```python
from build123d import *

# Parameters (mm, degrees)
F0_R     = 5
F0_R_2   = 4
F0_R_3   = 2.1
F1_DEPTH = 8
F2_DEPTH = 25
F3_R     = 4
F3_R_2   = 2.1
F4_DEPTH = 4
F5_DEPTH = 6
F6_DEPTH = 1
F7_R     = 0.5


with BuildPart() as f1:
    # F0 (on Top) → F1 (new body)
    with BuildSketch(Plane.XY):
        with BuildLine():
            ThreePointArc((-96.161356, -13.406398), (-102.161356, -19.406398), (-96.161356, -25.406398))
            Line((-96.161356, -25.406398), (-46.161356, -25.406398))
            ThreePointArc((-46.161356, -25.406398), (-40.161356, -19.406398), (-46.161356, -13.406398))
            Line((-46.161356, -13.406398), (-96.161356, -13.406398))
        make_face()
        with BuildLine():
            Line((-96.161356, -13.906398), (-46.161356, -13.906398))
            ThreePointArc((-46.161356, -13.906398), (-40.661356, -19.406398), (-46.161356, -24.906398))
            Line((-46.161356, -24.906398), (-96.161356, -24.906398))
            ThreePointArc((-96.161356, -24.906398), (-101.661356, -19.406398), (-96.161356, -13.906398))
        make_face(mode=Mode.SUBTRACT)
        with BuildLine():
            ThreePointArc((-46.161356, -24.906398), (-40.661356, -19.406398), (-46.161356, -13.906398))
            Line((-46.161356, -13.906398), (-96.161356, -13.906398))
            ThreePointArc((-96.161356, -13.906398), (-101.661356, -19.406398), (-96.161356, -24.906398))
            Line((-96.161356, -24.906398), (-46.161356, -24.906398))
        make_face()
        with Locations((-96.161356, -19.406398)):
            Circle(F0_R, mode=Mode.SUBTRACT)
        with BuildLine():
            ThreePointArc((-85.161356, -22.406398), (-88.161356, -19.406398), (-85.161356, -16.406398))
            Line((-85.161356, -16.406398), (-57.161356, -16.406398))
            ThreePointArc((-57.161356, -16.406398), (-54.161356, -19.406398), (-57.161356, -22.406398))
            Line((-57.161356, -22.406398), (-85.161356, -22.406398))
        make_face(mode=Mode.SUBTRACT)
        with Locations((-46.161356, -19.406398)):
            Circle(F0_R, mode=Mode.SUBTRACT)
        with Locations((-96.161356, -19.406398)):
            Circle(F0_R)
        with Locations((-96.161356, -19.406398)):
            Circle(F0_R_2, mode=Mode.SUBTRACT)
        with Locations((-96.161356, -19.406398)):
            Circle(F0_R_2)
        with Locations((-96.161356, -19.406398)):
            Circle(F0_R_3, mode=Mode.SUBTRACT)
        with Locations((-96.161356, -19.406398)):
            Circle(F0_R_3)
        with BuildLine():
            Line((-57.161356, -16.406398), (-85.161356, -16.406398))
            ThreePointArc((-85.161356, -16.406398), (-88.161356, -19.406398), (-85.161356, -22.406398))
            Line((-85.161356, -22.406398), (-57.161356, -22.406398))
            ThreePointArc((-57.161356, -22.406398), (-54.161356, -19.406398), (-57.161356, -16.406398))
        make_face()
        with Locations((-46.161356, -19.406398)):
            Circle(F0_R)
        with Locations((-46.161356, -19.406398)):
            Circle(F0_R_2, mode=Mode.SUBTRACT)
        with Locations((-46.161356, -19.406398)):
            Circle(F0_R_2)
        with Locations((-46.161356, -19.406398)):
            Circle(F0_R_3, mode=Mode.SUBTRACT)
        with Locations((-46.161356, -19.406398)):
            Circle(F0_R_3)
    extrude(amount=F1_DEPTH)

    # F0 (on Top) → F2 (cut)
    with BuildSketch(Plane.XY):
        with Locations((-96.161356, -19.406398)):
            Circle(F0_R_3)
        with Locations((-46.161356, -19.406398)):
            Circle(F0_R_3)
    extrude(amount=F2_DEPTH, mode=Mode.SUBTRACT)

    # F3 (on face) → F4 (cut)
    with BuildSketch(Plane.XY.offset(8)):
        with Locations((-96.161356, -19.406398)):
            Circle(F3_R)
        with Locations((-96.161356, -19.406398)):
            Circle(F3_R_2, mode=Mode.SUBTRACT)
        with Locations((-46.161356, -19.406398)):
            Circle(F3_R)
        with Locations((-46.161356, -19.406398)):
            Circle(F3_R_2, mode=Mode.SUBTRACT)
    extrude(amount=-F4_DEPTH, mode=Mode.SUBTRACT)

    # F0 (on Top) → F5 (cut)
    with BuildSketch(Plane.XY):
        with BuildLine():
            Line((-57.161356, -16.406398), (-85.161356, -16.406398))
            ThreePointArc((-85.161356, -16.406398), (-88.161356, -19.406398), (-85.161356, -22.406398))
            Line((-85.161356, -22.406398), (-57.161356, -22.406398))
            ThreePointArc((-57.161356, -22.406398), (-54.161356, -19.406398), (-57.161356, -16.406398))
        make_face()
    extrude(amount=F5_DEPTH, mode=Mode.SUBTRACT)

    # F0 (on Top) → F6 (cut)
    with BuildSketch(Plane.XY):
        with Locations((-96.161356, -19.406398)):
            Circle(F0_R)
        with Locations((-96.161356, -19.406398)):
            Circle(F0_R_2, mode=Mode.SUBTRACT)
        with Locations((-96.161356, -19.406398)):
            Circle(F0_R_2)
        with Locations((-96.161356, -19.406398)):
            Circle(F0_R_3, mode=Mode.SUBTRACT)
        with Locations((-46.161356, -19.406398)):
            Circle(F0_R)
        with Locations((-46.161356, -19.406398)):
            Circle(F0_R_2, mode=Mode.SUBTRACT)
        with Locations((-46.161356, -19.406398)):
            Circle(F0_R_2)
        with Locations((-46.161356, -19.406398)):
            Circle(F0_R_3, mode=Mode.SUBTRACT)
    extrude(amount=F6_DEPTH, mode=Mode.SUBTRACT)

    # F7
    f7_edges = [f1.edges().sort_by_distance(p)[0] for p in [
        (-71.161356, -25.406398, 8),
    ]]
    fillet(f7_edges, radius=F7_R)


solid = f1.part
```
Design review of the part built by this model. Coordinates are the model's own, in mm. A direction names the side the tool comes from. Coordinates: 2 decimals unless noted, no trailing zeros. Order: outer loops, then holes, each group sorted by start corner. A loop starts at its lowest first (then second) coordinate and runs counter-clockwise, first axis right, second up. Notation, with made-up numbers: M 80.25,80 L 103.25,80 A20 ccw 103.25,117 Z; hole C 47,60 d4. An arc over 180 degrees is marked long. Answer as a JSON object with one key per item and string values. Group by question number.
1) Tool access review of faces 1 (the flat face through (-96, -22, 1)), 2 (the cylindrical face through (-40.163, -19.538, 3.698)), 3 (the flat face through (-44, -21, 4)): name each direction out of +Z, -Z, +X, -X, +Y, -Y from which nothing blocks a thin tool from reaching the whole face with its end or side.
2) For pin 1 (3 mm diameter, centred on x = -71, y = -18.5, fed in from -Z); pin 2 (2.5 mm diameter, centred on x = -96.16, y = -19.41, fed in from +Z); pin 3 (4 mm diameter, centred on x = -96, y = -19, fed in from +Z); pin 4 (1 mm diameter, centred on y = -16.5, z = 4.5, fed in from +X), all flat-tipped, find the tip position at first contact; note any pin that passes through.
3) Add section A-A, the plane x = -47. Write out the cut boundary in (y, z), then the cut area to 3 significant figures.
4) Wall thickness on L1, parallel to Y at x = -72.5, z = 4.25; L2, parallel to X at y = -20.25, z = 3.5; L3, parallel to X at y = -16, z = 0.5: over which ranges is each line inside the solid? List them lowest first.
5) Add section B-B, the plane x = -73. Write out the cut boundary in (y, z).
6) Add section C-C, the plane z = 3. Write out the cut boundary in (x, y), then the cut area to 3 significant figures.
Computed values:
{
 "1": {"face 1": "-Z", "face 2": "+Z, -Z, +X", "face 3": "+Z"},
 "2": {"pin 1": "stops at z = 6", "pin 2": "passes through", "pin 3": "stops at z = 4", "pin 4": "stops at x = -40.67"},
 "3": {"outline": "M -25.41,0 L -24.34,0 L -24.34,1 L -21.33,1 L -21.33,4 L -23.32,4 L -23.32,8 L -24.91,8 A0.5 ccw -25.41,7.5 Z; M -17.48,1 L -14.48,1 L -14.48,0 L -13.41,0 L -13.41,7.5 A0.5 ccw -13.91,8 L -15.5,8 L -15.5,4 L -17.48,4 Z", "area": "43.2 mm^2"},
 "4": {"L1": "y = -25.41 to -22.41, -16.41 to -13.41", "L2": "x = -102.1 to -98.08, -94.24 to -88.04, -54.28 to -48.08, -44.24 to -40.22", "L3": "x = -101.1 to -99.82, -92.5 to -49.82, -42.5 to -41.22"},
 "5": {"outline": "M -25.41,0 L -22.41,0 L -22.41,6 L -16.41,6 L -16.41,0 L -13.41,0 L -13.41,7.5 A0.5 ccw -13.91,8 L -24.91,8 A0.5 ccw -25.41,7.5 Z"},
 "6": {"outline": "M -96.16,-25.41 L -46.16,-25.41 A6 ccw -46.16,-13.41 L -96.16,-13.41 A6 ccw Z; hole C -96.16,-19.41 d4.2; hole M -85.16,-22.41 L -57.16,-22.41 A3 ccw -57.16,-16.41 L -85.16,-16.41 A3 ccw Z; hole C -46.16,-19.41 d4.2", "area": "489 mm^2"}
}
